Autodesk Inventor part; units mm, degrees
ref_plane "YZ Plane" through (0, 0, 0) normal (1, 0, 0) x (0, 1, 0)
ref_plane "XZ Plane" through (0, 0, 0) normal (0, 1, 0) x (-1, 0, 0)
ref_plane "XY Plane" through (0, 0, 0) normal (0, 0, 1) x (1, 0, 0)
sketch "Sketch2" plane through (0, 0, 0) normal (0, 1, 0) x (-1, 0, 0)
  line L0 (-2.5, 6) -> (2.5, 6)
  line L1 (2.5, 6) -> (2.5, -6)
  line L2 (2.5, -6) -> (-2.5, -6)
  line L3 (-2.5, -6) -> (-2.5, 6)
  line L4 (-2.5, 6) -> (2.5, -6) construction
  line L5 (2.5, 6) -> (-2.5, -6) construction
  line L6 (-5.5, 9) -> (5.5, 9)
  line L7 (5.5, 9) -> (5.5, -9)
  line L8 (5.5, -9) -> (-5.5, -9)
  line L9 (-5.5, -9) -> (-5.5, 9)
  line L10 (-5.5, 9) -> (5.5, -9) construction
  line L11 (5.5, 9) -> (-5.5, -9) construction
  line L12 (-2.5, 0) -> (2.5, 0)
  circle A0 centre (0, -3) radius 0.9
  circle A1 centre (0, 3) radius 0.9
  point P0 (0, 0)
  dimension "d2" = 5
  dimension "d3" = 12
  dimension "d4" = 11
  dimension "d5" = 18
  dimension "d13" = 1.8
  dimension "d14" = 2.5
  dimension "d15" = 3
extrude "Extrusion2" add sketch "Sketch2" along normal blind 4 contours L6 L7 L8 L9
sketch "Sketch3" plane through (0, 4, 0) normal (0, 1, 0) x (1, 0, 0)
  line L0 (-2.5, 6) -> (2.5, 6)
  line L1 (2.5, -6) -> (-2.5, -6)
  line L2 (-2.5, -6) -> (-2.5, 6)
  line L3 (-2.5, 6) -> (2.5, 6)
  line L4 (2.5, 6) -> (2.5, -6)
  line L5 (2.5, -6) -> (-2.5, 6) construction
  line L6 (-2.5, -6) -> (2.5, 6) construction
  line L7 (5.5, 9) -> (-5.5, 9)
  line L8 (-5.5, 9) -> (-5.5, -9)
  line L9 (-5.5, -9) -> (5.5, -9)
  line L10 (5.5, -9) -> (5.5, 9)
  line L11 (5.5, 9) -> (-5.5, -9) construction
  line L12 (-5.5, 9) -> (5.5, -9) construction
  line L13 (2.5, -6) -> (5.5, -6)
  line L14 (2.5, 6) -> (5.5, 6)
  point P0 (0, 0)
extrude "Extrusion3" add sketch "Sketch3" along normal blind 3 contours L2 L1 L13 L10 L9 L8 L7 L14 L0
sketch "Sketch4" plane through (0, 7, 0) normal (0, 1, 0) x (1, 0, 0)
  line L0 (5.5, 9) -> (-5.5, 9)
  line L1 (5.5, -9) -> (-5.5, -9)
  line L2 (-5.5, -9) -> (-5.5, 9)
  line L3 (-5.5, 9) -> (5.5, 9)
  line L4 (5.5, 9) -> (5.5, -9)
  line L5 (5.5, -9) -> (-5.5, 9) construction
  line L6 (-5.5, -9) -> (5.5, 9) construction
  point P0 (0, 0)
extrude "Extrusion4" add sketch "Sketch4" along normal blind 2
extrude "Extrusion5" cut sketch "Sketch2" along normal through all contours A0 | A1
properties part number "pokus"
Design review of the part built by this model. Coordinates are the model's own, in mm. A direction names the side the tool comes from. Give positions to 0.01 mm unless a question says otherwise; leave off trailing zeros. Loops run counter-clockwise (first coordinate to the right, second up) from the corner with the lowest first, then second, coordinate; pieces in that order, holes last. Notation, with made-up numbers: (14, 70.5) - (56, 70.5) arc R10 cw to (56, 79.5) - close; hole circle Ø11 at (-33.75, 23). An arc over 180 degrees is marked (long way). Use CSV: the item, a comma, the result in double quotes. Start each with the question number.
1. Machinability: for faces 1 (the flat face through (-2.5, 3, 0)), 2 (the flat face through (1, 7, 0)), 3 (the flat face through (1, 3, -6)), which of the approach directions +Z, -Z, +X, -X, +Y, -Y give a long, thin tool a straight path to every point of the face, cutting with its end or side? Answer none if there is none.
2. Add section A-A (z = 4.25). State the section outline as (x, y) points.
3. Add section D-D (y = 4.75). State the section outline as (x, z) points.
4. Add section B-B (y = 2.5). State the section outline as (x, z) points.
5. Add section C-C (x = 0). State the section outline as (y, z) points.
6. Draft analysis for pull direction Z (two halves, no side actions). For faces 4 (the flat face through (0, 4, -9)), 5 (the flat face through (4, 4, 0)), 6 (the flat face through (5.5, 3, 0)), state which applies: released by +Z, released by -Z, zero draft, split by the parting line, or undercut.
7. Wall thickness on L1, parallel to Z at x = 0, y = 8.2; L2, parallel to Z at x = -1.5, y = 0.75; L3, parallel to X at y = 3, z = -4.25: over which ranges is each line inside the solid? List them lowest first.
8. Insertion check: P1, Ø1.4, axis at x = 0, z = 3, coming from the -Y side; P2, Ø2.5, axis at x = 1, z = -2, coming from the -Y side. Each pin has a flat end and moves straight along its axis. Give the tip position at first contact, or say it passes through.
Results found:
1,face 1,"-Y"
1,face 2,"+X"
1,face 3,"none"
2,outline,"(-5.5, 0) - (-2.5, 0) - (-2.5, 7) - (5.5, 7) - (5.5, 9) - (-5.5, 9) - close; (2.5, 0) - (5.5, 0) - (5.5, 4) - (2.5, 4) - close"
3,outline,"(-5.5, -9) - (5.5, -9) - (5.5, -6) - (-2.5, -6) - (-2.5, 6) - (5.5, 6) - (5.5, 9) - (-5.5, 9) - close"
4,outline,"(-5.5, -9) - (5.5, -9) - (5.5, 9) - (-5.5, 9) - close; hole (-2.5, -6) - (2.5, -6) - (2.5, 6) - (-2.5, 6) - close"
5,outline,"(0, -9) - (9, -9) - (9, -3.9) - (7, -3.9) - (7, -6) - (0, -6) - close; (0, 6) - (7, 6) - (7, 3.9) - (9, 3.9) - (9, 9) - (0, 9) - close; (7, -2.1) - (9, -2.1) - (9, 2.1) - (7, 2.1) - close"
6,face 4,"released by -Z"
6,face 5,"undercut"
6,face 6,"zero draft"
7,L1,"z = -9 to -3.9, -2.1 to 2.1, 3.9 to 9"
7,L2,"z = -9 to -6, 6 to 9"
7,L3,"x = -5.5 to -2.5, 2.5 to 5.5"
8,P1,"passes through"
8,P2,"stops at y = 7"
